Could you check a few things on this model? Use its own coordinates, in mm. A direction names the side the tool comes from. Round coordinates to 2 decimals unless told otherwise and drop trailing zeros. Loops run counter-clockwise (first coordinate to the right, second up) from the corner with the lowest first, then second, coordinate; pieces in that order, holes last. Notation, with made-up numbers: M 72.5,47 L 124.5,47 A20 ccw 124.5,70 Z; hole C 86.5,44 d10. An arc over 180 degrees is marked long. Answer in a Markdown table with one row per item.
```python
from build123d import *

# Parameters (mm, degrees)
BOSS_EXTRUDE1_DEPTH = 34.5
BOSS_EXTRUDE2_DEPTH = 24


with BuildPart() as part:
    # Sketch2 → Boss-Extrude1 (new body)
    with BuildSketch(Plane.XY):
        with BuildLine():
            Line((-9, 3), (9, 3))
            Line((9, 3), (9, -1))
            Line((9, -1), (8.394427191, -1.302786405))
            ThreePointArc((8.394427191, -1.302786405), (8.118033989, -1.75), (8.394427191, -2.197213595))
            Line((8.394427191, -2.197213595), (9, -2.5))
            Line((9, -2.5), (9, -3))
            Line((9, -3), (12, -3))
            Line((12, -3), (12, 6))
            Line((12, 6), (-12, 6))
            Line((-12, 6), (-12, -3))
            Line((-12, -3), (-9, -3))
            Line((-9, -3), (-9, -2.5))
            Line((-9, -2.5), (-8.394427191, -2.197213595))
            ThreePointArc((-8.394427191, -2.197213595), (-8.118033989, -1.75), (-8.394427191, -1.302786405))
            Line((-8.394427191, -1.302786405), (-9, -1))
            Line((-9, -1), (-9, 3))
        make_face()
    extrude(amount=BOSS_EXTRUDE1_DEPTH)

    # Sketch3 → Boss-Extrude2 (add)
    with BuildSketch(Plane.ZY.offset(12)):
        Polygon((29.947523085, 35.6), (30.247523085, 10), (4.047523085, 10), (4.347523085, 35.4), (0.347802057, 35.4472408), (0, 6), (34.5, 6), (34.152547528, 35.64927763), align=None)
    extrude(amount=-BOSS_EXTRUDE2_DEPTH)


solid = part.part
```
1) I need wall thicknesses on line 1 (Y direction, x = -10.25, z = 29); line 2 (X direction, y = 2.5, z = 19); line 3 (Z direction, x = 10.5, y = 7). Which ranges of each line are inside material? Lowest first, please.
Computed:
| item | result |
|---|---|
| line 1 | y = -3 to 10 |
| line 2 | x = -12 to -9, 9 to 12 |
| line 3 | z = 0.01 to 34.49 |
2) I want a section at B-B, the plane x = 4.5. Please give me the cut outline in (y, z), plus the area to 3 significant figures.
Computed:
| item | result |
|---|---|
| outline | M 3,0 L 6,0 L 35.45,0.35 L 35.4,4.35 L 10,4.05 L 10,30.25 L 35.6,29.95 L 35.65,34.15 L 6,34.5 L 3,34.5 Z |
| area | 451 mm² |
3) Which directions (+Z, -Z, +X, -X, +Y, -Y) give clear straight access to the entire face, cutting with the end or side of a thin tool? Please do faces 4 (the face through (-11, -3, 17)), 5 (the face through (-8.12, -1.76, 17.01)).
Computed:
| item | result |
|---|---|
| face 4 | +Z, -Z, +X, -X, -Y |
| face 5 | +Z, -Z |
4) I want a section at C-C, the plane z = 14. Please give me the cut outline in (x, y), plus the area to 3 significant figures.
Computed:
| item | result |
|---|---|
| outline | M -12,-3 L -9,-3 L -9,-2.5 L -8.39,-2.2 A0.5 ccw -8.39,-1.3 L -9,-1 L -9,3 L 9,3 L 9,-1 L 8.39,-1.3 A0.5 ccw 8.39,-2.2 L 9,-2.5 L 9,-3 L 12,-3 L 12,10 L -12,10 Z |
| area | 206 mm² |
5) Will these pins go through, and if not, where does the flat tip stop? P1, Ø2, axis at x = -4, y = 13.5, coming from the -Z side; P2, Ø12, axis at x = 8.5, z = 24, coming from the +Y side; P3, Ø5, axis at x = -1, z = 11.5, coming from the +Y side; P4, Ø12, axis at y = 19.5, z = 12.5, coming from the +X side.
Computed:
| item | result |
|---|---|
| P1 | stops at z = 0.08 |
| P2 | stops at y = 35.6 |
| P3 | stops at y = 10 |
| P4 | passes through |
6) If we mould it in two halves opening along Z, with no side actions, what happens to faces 1 (the face through (0, 10, 17)), 2 (the face through (0, 3, 17)), 3 (the face through (0, 4, 34.5))? For each: released by +Z, released by -Z, zero draft, split by the parting line, or undercut.
Computed:
| item | result |
|---|---|
| face 1 | undercut |
| face 2 | zero draft |
| face 3 | released by +Z |
7) I want a section at A-A, the plane y = 13. Please give me the cut outline in (x, z).
Computed:
| item | result |
|---|---|
| outline | M -12,0.08 L 12,0.08 L 12,4.08 L -12,4.08 Z; M -12,30.21 L 12,30.21 L 12,34.42 L -12,34.42 Z |
